```python
from build123d import *

# Parameters (mm, degrees)
SKETCH1_W                 = 350
SKETCH1_H                 = 250
BOSS_EXTRUDE1_DEPTH       = 26
SKETCH2_W                 = 1
SKETCH2_H                 = 40
BOSS_EXTRUDE2_DEPTH       = 50
M48_CLEARANCE_HOLE1_D     = 55
M48_CLEARANCE_HOLE1_DEPTH = 13
FILLET1_R                 = 150


with BuildPart() as part:
    # Sketch1 → Boss-Extrude1 (new body)
    with BuildSketch(Plane.XY.offset(26)):
        with Locations((175, 125)):
            Rectangle(SKETCH1_W, SKETCH1_H)
    extrude(amount=-BOSS_EXTRUDE1_DEPTH)

    # Sketch2 → Boss-Extrude2 (add)
    with BuildSketch(Plane(origin=(0, 0, 0), x_dir=(-1, 0, 0), z_dir=(0, 0, -1))):
        with Locations((-279.5, 30)):
            Rectangle(SKETCH2_W, SKETCH2_H)
    extrude(amount=BOSS_EXTRUDE2_DEPTH)

    # M48 Clearance Hole1
    with Locations(Plane.XY.offset(26)):
        with Locations((55, 80), (212.082039325, 194.126781955), (272.082039325, 150.534230275), (295, 80), (137.917960675, 194.126781955), (77.917960675, 150.534230275)):
            Hole(M48_CLEARANCE_HOLE1_D / 2, depth=M48_CLEARANCE_HOLE1_DEPTH)

    # Fillet1
    fillet1_edges = [part.edges().sort_by_distance(p)[0] for p in [
        (0, 250, 13),
        (350, 250, 13),
    ]]
    fillet(fillet1_edges, radius=FILLET1_R)


solid = part.part
```
Input: part model. Units: mm. Frame: model coordinates. A direction names the side the tool comes from. Coordinates: 2 decimals unless noted, no trailing zeros. Write each loop counter-clockwise with the first axis right and the second up, starting at its lowest first coordinate (ties: lowest second). Pieces come first, ordered by that corner, then holes.
1) Section D-D on z = -33.5. Output: boundary loops of the cut face in (x, y).
2) Section B-B on z = 20.5. Output: boundary loops of the cut face in (x, y).
3) Section A-A on y = 80. Output: boundary loops of the cut face in (x, z), and give its area (3 significant figures).
4) Material intervals for line 1 along X through (y, z) = (26, -46.5); line 2 along Z through (x, y) = (246.5, 45); line 3 along Z through (x, y) = (280, 141.5), sorted ascending.
5) Mould query, pull axis Y, two halves, no side actions, for faces 4 (the cylindrical face through (232.351, 212.713, 19.409)), 5 (the flat face through (280, 30, -25)), 6 (the cylindrical face through (42.77, 204.89, 12.82)). Classes: pulls with the +Y half, pulls with the -Y half, needs draft (parallel to the pull), parting line crosses it, or undercut.
6) Set-up query: faces 1 (the flat face through (279, 30, -25)), 2 (the flat face through (272, 151, 13)), 3 (the cylindrical face through (304.89, 207.23, 12.82)). Return all of +Z, -Z, +X, -X, +Y, -Y with unobstructed straight access to the full face (end or side cutting, diameter ignored); none if empty.
7) Section C-C on x = 295. Output: boundary loops of the cut face in (y, z).
8) Pin query (flat end, axial travel): pin 1 Ø1 at (x, z) = (210.5, 3) entering from -Y; pin 2 Ø5 at (x, y) = (230, 121.5) entering from -Z; pin 3 Ø16.5 at (x, y) = (264.5, 142) entering from +Z; pin 4 Ø0.5 at (x, z) = (279.5, -23.5) entering from +Y. Return the tip coordinate at first contact, or that it passes through.
Check result:
1. outline: (279, 10) - (280, 10) - (280, 50) - (279, 50) - close
2. outline: (0, 0) - (350, 0) - (350, 100) arc R150 ccw to (200, 250) - (150, 250) arc R150 ccw to (0, 100) - close; hole circle Ø55 at (55, 80); hole circle Ø55 at (77.92, 150.53); hole circle Ø55 at (137.92, 194.13); hole circle Ø55 at (212.08, 194.13); hole circle Ø55 at (272.08, 150.53); hole circle Ø55 at (295, 80)
3. outline: (0, 0) - (350, 0) - (350, 26) - (322.5, 26) - (322.5, 13) - (267.5, 13) - (267.5, 26) - (82.5, 26) - (82.5, 13) - (27.5, 13) - (27.5, 26) - (0, 26) - close
3. area: 7,670 mm2
4. line 1: x = 279 to 280
4. line 2: z = 0 to 26
4. line 3: z = 0 to 13
5. face 4: undercut
5. face 5: needs draft
5. face 6: pulls with the +Y half
6. face 1: -Z, -X, +Y, -Y
6. face 2: +Z
6. face 3: +Z, -Z, +X, +Y
7. outline: (0, 0) - (216.08, 0) - (216.08, 26) - (165.73, 26) - (165.73, 13) - (135.33, 13) - (135.33, 26) - (107.5, 26) - (107.5, 13) - (52.5, 13) - (52.5, 26) - (0, 26) - close
8. pin 1: stops at y = 0
8. pin 2: stops at z = 0
8. pin 3: stops at z = 13
8. pin 4: stops at y = 50
